from build123d import *

# Parameters (mm, degrees)
SKETCH1_R           = 4.5
BOSS_EXTRUDE1_DEPTH = 10
BOSS_EXTRUDE2_START = 2
SKETCH2_R           = 7.5
BOSS_EXTRUDE2_DEPTH = 2
SKETCH3_R           = 4.5
BOSS_EXTRUDE3_DEPTH = 25
BOSS_EXTRUDE4_DEPTH = 10
SKETCH5_R           = 2
CUT_EXTRUDE1_DEPTH  = 6


with BuildPart() as part:
    # Sketch1 → Boss-Extrude1 (new body)
    with BuildSketch(Plane.XY):
        Circle(SKETCH1_R)
        with BuildLine():
            Line((-1.85, 1.966596044), (-1.85, -1.966596044))
            ThreePointArc((-1.85, -1.966596044), (0, -2.7), (1.85, -1.966596044))
            Line((1.85, -1.966596044), (1.85, 1.966596044))
            ThreePointArc((1.85, 1.966596044), (1.851058142, 1.9656001), (1.852115749, 1.964603587))
            ThreePointArc((1.852115749, 1.964603587), (0.001453124, 2.699999609), (-1.85, 1.966596044))
        make_face(mode=Mode.SUBTRACT)
    extrude(amount=BOSS_EXTRUDE1_DEPTH)

    # Sketch2 → Boss-Extrude2 (add)
    with BuildSketch(Plane(origin=(0, 0, 0), x_dir=(-1, 0, 0), z_dir=(0, 0, -1)).offset(BOSS_EXTRUDE2_START)):
        Circle(SKETCH2_R)
        with BuildLine():
            Line((1.85, 1.966596044), (1.85, -1.966596044))
            ThreePointArc((1.85, -1.966596044), (0, -2.7), (-1.85, -1.966596044))
            Line((-1.85, -1.966596044), (-1.85, 1.966596044))
            ThreePointArc((-1.85, 1.966596044), (0, 2.7), (1.85, 1.966596044))
        make_face(mode=Mode.SUBTRACT)
    extrude(amount=-BOSS_EXTRUDE2_DEPTH)

    # Sketch3 → Boss-Extrude3 (add)
    with BuildSketch(Plane.XY.offset(10)):
        Circle(SKETCH3_R)
    extrude(amount=BOSS_EXTRUDE3_DEPTH)

    # Sketch4 → Boss-Extrude4 (add)
    with BuildSketch(Plane.XY.offset(35)):
        Polygon((1.920788906, 4.069468022), (-2.563868233, 3.698185999), (-4.48465714, -0.371282023), (-1.920788906, -4.069468022), (2.563868233, -3.698185999), (4.48465714, 0.371282023), align=None)
    extrude(amount=BOSS_EXTRUDE4_DEPTH)

    # Sketch5 → Cut-Extrude1 (cut)
    with BuildSketch(Plane.XY.offset(45)):
        Circle(SKETCH5_R)
    extrude(amount=-CUT_EXTRUDE1_DEPTH, mode=Mode.SUBTRACT)


solid = part.part
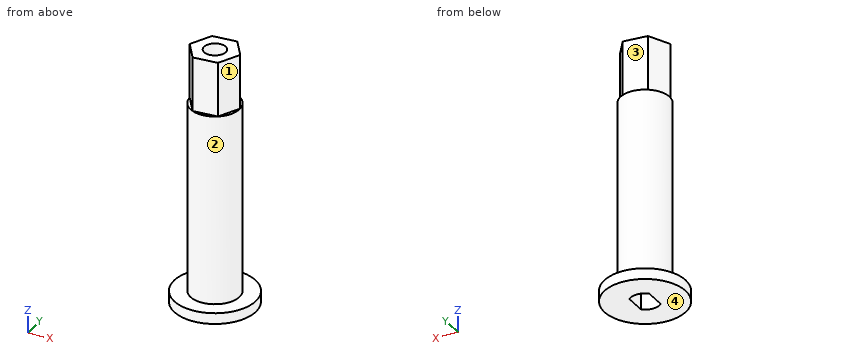
Input: part model. Units: mm. Frame: model coordinates. Face numbers are marked on the shaded views. A direction names the side the tool comes from. Give positions to 0.01 mm unless a question says otherwise; leave off trailing zeros. Write each loop counter-clockwise with the first axis right and the second up, starting at its lowest first coordinate (ties: lowest second). Pieces come first, ordered by that corner, then holes.
Q1. Section D-D, the plane y = 6. Output: boundary loops of the cut face in (x, z), plus the area to 3 significant figures.
Q2. First-contact query: P1, Ø2, axis at x = 3, z = 14.5, coming from the -Y side; P2, Ø4, axis at y = 5.5, z = 36, coming from the +X side; P3, Ø0.6, axis at x = 0.5, y = 4.5, coming from the +Z side; P4, Ø1, axis at x = 6, z = 36.5, coming from the +Y side. Flat tips, straight axial feed; report the tip coordinate or a pass-through.
Q3. Set-up query: the marked faces 1, 2, 3 and 4. Return all of +Z, -Z, +X, -X, +Y, -Y with unobstructed straight access to the full face (end or side cutting, diameter ignored); none if empty.
Q4. Material intervals for probe 1 along Z at (x, y) = (5, -2.5); probe 2 along X at (y, z) = (0.5, 41.5); probe 3 along Z at (x, y) = (-0.5, 2.25), sorted ascending.
Q5. Section A-A, the plane z = 6. Output: boundary loops of the cut face in (x, y).
Q6. Section C-C, the plane z = 37. Output: boundary loops of the cut face in (x, y).
Q7. Section B-B, the plane x = 0. Output: boundary loops of the cut face in (y, z).
Filled in:
1. outline: (-4.5, -2) - (4.5, -2) - (4.5, 0) - (-4.5, 0) - close
1. area: 18.0 mm2
2. P1: stops at y = -4.03
2. P2: stops at x = 2.46
2. P3: stops at z = 35
2. P4: passes through
3. face 1: +Z, +X, -Y
3. face 2: +Z
3. face 3: +Z, -X, +Y
3. face 4: -Z, +X, -X, +Y, -Y
4. probe 1: z = -2 to 0
4. probe 2: x = -4.07 to -1.94, 1.94 to 4.4
4. probe 3: z = 10 to 45
5. outline: circle Ø9 at (0, 0); hole (-1.85, -1.97) arc R2.7 ccw to (1.85, -1.97) - (1.85, 1.97) arc R2.7 ccw to (-1.85, 1.97) - close
6. outline: (-4.48, -0.37) - (-1.92, -4.07) - (2.56, -3.7) - (4.48, 0.37) - (1.92, 4.07) - (-2.56, 3.7) - close
7. outline: (-7.5, -2) - (-2.7, -2) - (-2.7, 10) - (2.7, 10) - (2.7, -2) - (7.5, -2) - (7.5, 0) - (4.5, 0) - (4.5, 35) - (3.91, 35) - (3.91, 45) - (2, 45) - (2, 39) - (-2, 39) - (-2, 45) - (-3.91, 45) - (-3.91, 35) - (-4.5, 35) - (-4.5, 0) - (-7.5, 0) - close
